from build123d import *

# Parameters (mm, degrees)
BOSS_EXTRU_1_DEPTH           = 20
ENL_V_MAT_EXTRU_1_DEPTH      = 871
ENL_V_MAT_EXTRU_1_DEPTH_BACK = 792
ESQUISSE5_R                  = 5
ENL_V_MAT_EXTRU_2_DEPTH      = 20
CONG_1_R                     = 10


with BuildPart() as part:
    # Esquisse1 → Boss.-Extru.1 (new body)
    with BuildSketch(Plane(origin=(0, 0, 0), x_dir=(0, 0, -1), z_dir=(1, 0, 0))):
        Polygon((635.709590149, 813.74559194), (-385.471678665, 529.511856746), (-776.290409851, -136.25440806), (-776.290409851, -573.25440806), (635.709590149, -573.25440806), align=None)
    extrude(amount=BOSS_EXTRU_1_DEPTH)

    # Esquisse4 → Enlèv. mat.-Extru.1 (cut, two sides: drawn at the far end of the back side and taken through both)
    with BuildSketch(Plane.XY.offset(-ENL_V_MAT_EXTRU_1_DEPTH_BACK)):
        Polygon((0, -573.25440806), (0, -571.922503428), (20, -573.25440806), align=None)
    extrude(amount=ENL_V_MAT_EXTRU_1_DEPTH + ENL_V_MAT_EXTRU_1_DEPTH_BACK, mode=Mode.SUBTRACT)

    # Esquisse5 → Enlèv. mat.-Extru.2 (cut)
    with BuildSketch(Plane(origin=(-37.919143048, -569.397269313, 0), x_dir=(0.9977898861170226, -0.06644804859873017, 0), z_dir=(-0.06644804859873017, -0.9977898861170226, 0))):
        with Locations((48.027434489, -625.709590149)):
            Circle(ESQUISSE5_R)
    extrude(amount=-ENL_V_MAT_EXTRU_2_DEPTH, mode=Mode.SUBTRACT)

    # Congé1
    cong_1_edges = [part.edges().sort_by_distance(p)[0] for p in [
        (0, 120.911544256, -635.709590149),
        (20, 120.24559194, -635.709590149),
    ]]
    fillet(cong_1_edges, radius=CONG_1_R - 0.0001)  # a hair under: the kernel refuses the full size


solid = part.part
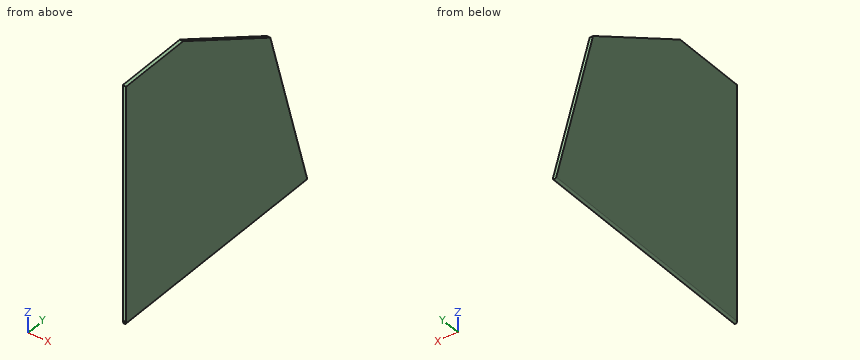
Can you work these out from the model? Positions are in its coordinate system, mm. Coordinates: 2 decimals unless noted, no trailing zeros. Write each loop counter-clockwise with the first axis right and the second up, starting at its lowest first coordinate (ties: lowest second). Pieces come first, ordered by that corner, then holes.
Q1. For P1, Ø6, axis at x = 5.5, z = 599, coming from the -Y side; P2, Ø12, axis at x = 13.5, y = -73, coming from the +Z side; P3, Ø1, axis at x = 5, y = -104.5, coming from the -Z side, each with a flat end and sliding along its axis, tell me the tip position at first contact or that it passes through.
Results found:
P1: stops at y = -572.49
P2: stops at z = 742.68
P3: stops at z = -634.64
Q2. Imagine slicing it at B-B, the plane z = -493. List the corners of the cut face in (x, y) for me, plus the area to 3 significant figures.
Results found:
outline: (0, -571.92) - (20, -573.25) - (20, 774.02) - (0, 774.02) - close
area: 26,900 mm2
Q3. Please list where these lines run through material, in increasing order: L1, parallel to Y at x = 11.5, z = 686.5; L2, parallel to Y at x = 14.5, z = 707; L3, parallel to Z at x = 14.5, y = 448.
Results found:
L1: y = -572.69 to 16.71
L2: y = -572.89 to -18.22
L3: z = -634.64 to 433.32
Q4. Imagine slicing it at C-C, the plane z = -117. List the corners of the cut face in (x, y) for me.
Results found:
outline: (0, -571.92) - (20, -573.25) - (20, 669.37) - (0, 669.37) - close
